Could you check a few things on this drawing? It's one solid part, dimensions in mm from its lowest x, y, z. A direction names the side the tool comes from. Give positions to 0.01 mm unless a question says otherwise; leave off trailing zeros. Loops run counter-clockwise (first coordinate to the right, second up) from the corner with the lowest first, then second, coordinate; pieces in that order, holes last. Notation, with made-up numbers: M 57.25,13 L 103.25,13 A32 cw 103.25,49 Z; hole C 45,-21.5 d2. An arc over 180 degrees is marked long. Answer in a Markdown table with one row per item. Add a question column.
1. Which directions (+Z, -Z, +X, -X, +Y, -Y) give clear straight access to the entire face, cutting with the end or side of a thin tool? Please do the marked faces 1, 2 and 3.
2. If we section it at A-A on z = 15: List the corners of the cut face in (x, y) for me.
3. I'm going to push flat-ended pins straight in: pin 1 Ø4 at (y, z) = (8.5, 3.5) entering from -X; pin 2 Ø1 at (y, z) = (15, 27) entering from -X; pin 3 Ø15 at (x, z) = (13.5, 10.5) entering from +Y; pin 4 Ø8 at (y, z) = (21, 8.5) entering from +X. Where does each tip first touch, or does it pass through?
4. If we section it at C-C on y = 26: List the corners of the cut face in (x, z) for me.
5. If we section it at D-D on x = 31: List the corners of the cut face in (y, z) for me.
6. If we section it at B-B on x = 55: List the corners of the cut face in (y, z) for me.
7. I need wall thicknesses on line 1 along X through (y, z) = (2, 25); line 2 along Y through (x, z) = (57.75, 15); line 3 along X through (y, z) = (34, 22). Which ranges of each line are inside material? Lowest first, please. Write a range as from..to.
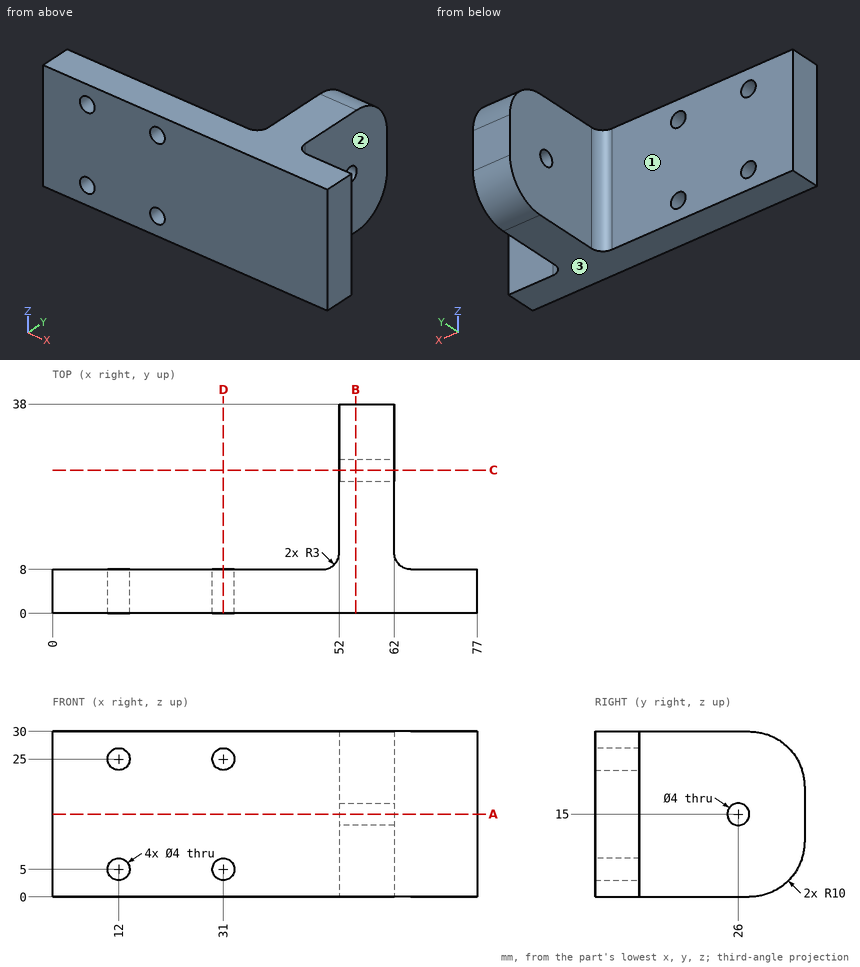
Results:
| question | item | result |
|---|---|---|
| 1 | face 1 | +Z, -Z, -X, +Y |
| 1 | face 2 | +Z, -Z, +X, +Y |
| 1 | face 3 | -Z, +X, -X, +Y, -Y |
| 2 | outline | M 0,0 L 77,0 L 77,8 L 65,8 A3 cw 62,11 L 62,24 L 52,24 L 52,11 A3 cw 49,8 L 0,8 Z; M 52,28 L 62,28 L 62,38 L 52,38 Z |
| 3 | pin 1 | x = 0 |
| 3 | pin 2 | x = 52 |
| 3 | pin 3 | y = 8 |
| 3 | pin 4 | x = 62 |
| 4 | outline | M 52,0 L 62,0 L 62,13 L 52,13 Z; M 52,17 L 62,17 L 62,30 L 52,30 Z |
| 5 | outline | M 0,0 L 8,0 L 8,3 L 0,3 Z; M 0,7 L 8,7 L 8,23 L 0,23 Z; M 0,27 L 8,27 L 8,30 L 0,30 Z |
| 6 | outline | M 0,0 L 28,0 A10 ccw 38,10 L 38,20 A10 ccw 28,30 L 0,30 Z; hole C 26,15 d4 |
| 7 | line 1 | 0..10, 14..29, 33..77 |
| 7 | line 2 | 0..24, 28..38 |
| 7 | line 3 | 52..62 |
